Check sheet for the modelled part. Datum: model origin and axes. Units: mm. Face numbers are marked on the shaded views. A direction names the side the tool comes from. Give positions to 0.01 mm unless a question says otherwise; leave off trailing zeros. Order: outer loops, then holes, each group sorted by start corner. A loop starts at its lowest first (then second) coordinate and runs counter-clockwise, first axis right, second up. Notation, with made-up numbers: (23.25, 65.5) - (74.25, 65.5) arc R8 cw to (74.25, 69.5) - close; hole circle Ø6 at (-34.5, -23). An arc over 180 degrees is marked (long way). Answer in a Markdown table with one row per item.
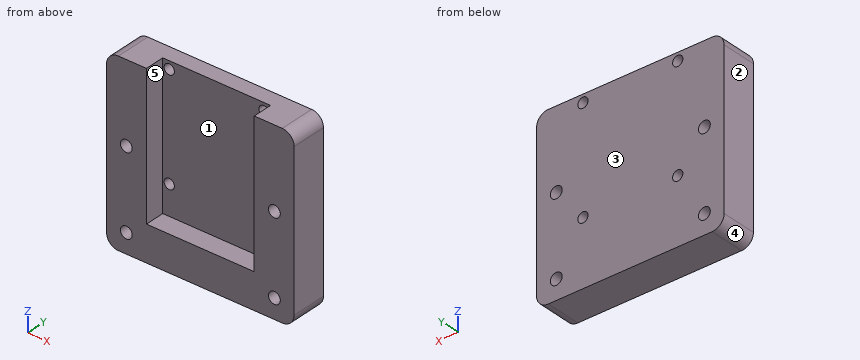
from build123d import *

# Parameters (mm, degrees)
SKETCH_1_W          = 47.5
SKETCH_1_H          = 45
SKETCH_1_R          = 1.5
SKETCH_1_R_2        = 1.3
EXTRUDE_1_DEPTH     = 9
SKETCH_2_W          = 27.3
SKETCH_2_H          = 36
CUT_EXTRUDE_1_DEPTH = 5
FILLET_1_R          = 3


with BuildPart() as part:
    # 草图1 → 凸台-拉伸1 (new body)
    with BuildSketch(Plane(origin=(0, 0, 0), x_dir=(1, 0, 0), z_dir=(0, 1, 0))):
        Rectangle(SKETCH_1_W, SKETCH_1_H)
        with Locations(Location((-18.75, 17.5, 0), (0, 0, 270))):
            Circle(SKETCH_1_R, mode=Mode.SUBTRACT)
        with Locations(Location((-18.75, -2.5, 0), (0, 0, 270))):
            Circle(SKETCH_1_R, mode=Mode.SUBTRACT)
        with Locations(Location((18.75, -2.5, 0), (0, 0, 90))):
            Circle(SKETCH_1_R, mode=Mode.SUBTRACT)
        with Locations(Location((18.75, 17.5, 0), (0, 0, 90))):
            Circle(SKETCH_1_R, mode=Mode.SUBTRACT)
        with Locations(Location((-12, -20.5, 0), (0, 0, 270))):
            Circle(SKETCH_1_R_2, mode=Mode.SUBTRACT)
        with Locations(Location((-12, 6, 0), (0, 0, 270))):
            Circle(SKETCH_1_R_2, mode=Mode.SUBTRACT)
        with Locations(Location((12, 6, 0), (0, 0, 90))):
            Circle(SKETCH_1_R_2, mode=Mode.SUBTRACT)
        with Locations(Location((12, -20.5, 0), (0, 0, 90))):
            Circle(SKETCH_1_R_2, mode=Mode.SUBTRACT)
    extrude(amount=EXTRUDE_1_DEPTH)

    # 草图2 → 切除-拉伸1 (cut)
    with BuildSketch(Plane.XZ):
        with Locations((0, 4.5)):
            Rectangle(SKETCH_2_W, SKETCH_2_H)
    extrude(amount=-CUT_EXTRUDE_1_DEPTH, mode=Mode.SUBTRACT)

    # 圆角1
    fillet_1_edges = [part.edges().sort_by_distance(p)[0] for p in [
        (23.75, 4.5, 22.5),
        (-23.75, 4.5, 22.5),
        (-23.75, 4.5, -22.5),
        (23.75, 4.5, -22.5),
    ]]
    fillet(fillet_1_edges, radius=FILLET_1_R)


solid = part.part
(1) Gauge pin test, flat ends, axial feed: P1, Ø8, axis at x = -3.5, z = 2.5, coming from the -Y side; P2, Ø2.5, axis at x = -6.5, y = 3, coming from the +Z side. Record the tip position at first contact, or that the pin passes through.
Geometry says:
| item | result |
|---|---|
| P1 | y = 5 |
| P2 | z = -13.5 |
(2) Thickness scan on L1, parallel to X at y = 7, z = 2.5; L2, parallel to Z at x = 12, y = 7.85; L3, parallel to X at y = 7.3, z = -6. Record the ranges inside material, lowest first.
Geometry says:
| item | result |
|---|---|
| L1 | -23.75 to -20.25, -17.25 to 17.25, 20.25 to 23.75 |
| L2 | -22.5 to -7.3, -4.7 to 19.2, 21.8 to 22.5 |
| L3 | -23.75 to -13.3, -10.7 to 10.7, 13.3 to 23.75 |
(3) Cross-section at C-C, the plane y = 5.75. Give the number of separate pieces and of enclosed holes in the cut face, then the cut area to 3 significant figures.
Geometry says:
| item | result |
|---|---|
| separate pieces | 1 |
| enclosed holes | 8 |
| area | 2,080 mm² |
(4) Cross-section at B-B, the plane x = -12. Record the cut outline in (y, z).
Geometry says:
| item | result |
|---|---|
| outline | (0, -22.5) - (9, -22.5) - (9, -7.3) - (5, -7.3) - (5, -13.5) - (0, -13.5) - close; (5, -4.7) - (9, -4.7) - (9, 19.2) - (5, 19.2) - close; (5, 21.8) - (9, 21.8) - (9, 22.5) - (5, 22.5) - close |
(5) Mould release check, pull along X, two halves, no side actions. Record for the marked faces 3, 4 and 5: pulls with the +X half, pulls with the -X half, needs draft (parallel to the pull), parting line crosses it, or undercut.
Geometry says:
| item | result |
|---|---|
| face 3 | needs draft |
| face 4 | pulls with the -X half |
| face 5 | undercut |
(6) Cross-section at A-A, the plane z = -17.5. Record the cut outline in (x, y), then the cut area to 4 significant figures.
Geometry says:
| item | result |
|---|---|
| outline | (-23.75, 0) - (-20.25, 0) - (-20.25, 9) - (-23.75, 9) - close; (-17.25, 0) - (17.25, 0) - (17.25, 9) - (-17.25, 9) - close; (20.25, 0) - (23.75, 0) - (23.75, 9) - (20.25, 9) - close |
| area | 373.5 mm² |
(7) Access from +Z, -Z, +X, -X, +Y, -Y to the whole of each face (thin tool, end or side, straight path). Record for the marked faces 1 and 2.
Geometry says:
| item | result |
|---|---|
| face 1 | +Z, -Y |
| face 2 | +Z, -Z, -X, +Y, -Y |
(8) Cross-section at D-D, the plane y = 3.25. Record the cut outline in (x, z), then the cut area to 3 significant figures.
Geometry says:
| item | result |
|---|---|
| outline | (-23.75, -19.5) arc R3 ccw to (-20.75, -22.5) - (20.75, -22.5) arc R3 ccw to (23.75, -19.5) - (23.75, 19.5) arc R3 ccw to (20.75, 22.5) - (13.65, 22.5) - (13.65, -13.5) - (-13.65, -13.5) - (-13.65, 22.5) - (-20.75, 22.5) arc R3 ccw to (-23.75, 19.5) - close; hole circle Ø3 at (-18.75, -17.5); hole circle Ø3 at (-18.75, 2.5); hole circle Ø3 at (18.75, -17.5); hole circle Ø3 at (18.75, 2.5) |
| area | 1,120 mm² |
